CAD build for the part. Positions are in the model's coordinates, mm. Face numbers are marked on the shaded views. A direction names the side the tool comes from. Coordinates: 2 decimals unless noted, no trailing zeros. Write each loop counter-clockwise with the first axis right and the second up, starting at its lowest first coordinate (ties: lowest second). Pieces come first, ordered by that corner, then holes. Notation, with made-up numbers: (-20.5, 61) - (11.5, 61) arc R27 ccw to (11.5, 78) - close; hole circle Ø5 at (62.25, 16). An arc over 180 degrees is marked (long way). Answer in a Markdown table with one row per item. Add a question column.
Q1. Band-saw the part on D-D (x = -16). List the corners of the cut face in (y, z).
Q2. Band-saw the part on A-A (y = -54). List the corners of the cut face in (x, z).
Q3. Drill centre lines: line 1 along Z through (x, y) = (25, 51); line 2 along Y through (x, z) = (-34, -65); line 3 along Y through (x, z) = (-35, -37). Where is each one in solid material? Low to high. Write a range as from..to.
Q4. 3-axis set-ups, long thin cutter, end or side, ignore diameter. For the marked faces 1 and 2: which of +Z, -Z, +X, -X, +Y, -Y reach the whole face in a straight line?
Q5. Band-saw the part on B-B (x = -39). List the corners of the cut face in (y, z).
Q6. Band-saw the part on C-C (z = -28.5). List the corners of the cut face in (x, y), and give its area (3 significant figures).
Q7. Pin check, flat tips, straight feed: pin 1 (6 mm diameter, centred on x = -14.5, y = -24, fed in from -Z); pin 2 (2.5 mm diameter, centred on x = 34.5, y = 59.5, fed in from -Z); pin 3 (3 mm diameter, centred on x = 29.5, z = -61.5, fed in from -Y); pin 4 (9.5 mm diameter, centred on x = -37, y = -56.5, fed in from -Z). Stop position of each tip, or through.
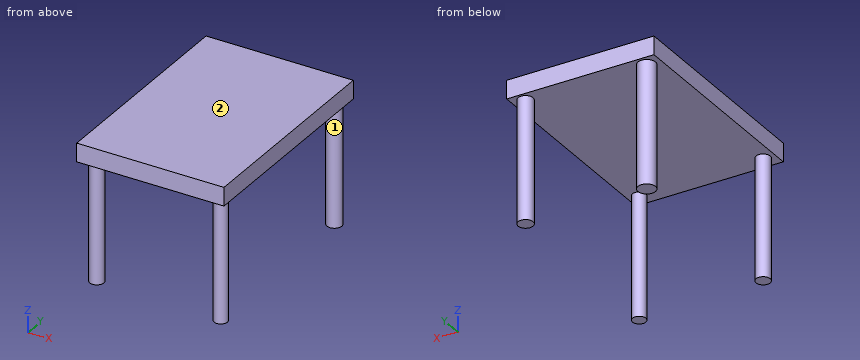
```python
from build123d import *

# Parameters (mm, degrees)
F0_W     = 89.114376
F0_H     = 129.904926
F1_DEPTH = 11.176
F2_R     = 5.277651
F6_DEPTH = 74.422
F3_R     = 4.552344
F7_DEPTH = 74.168
F4_R     = 4.294458
F8_DEPTH = 73.406
F5_R     = 4.020045
F9_DEPTH = 74.422


with BuildPart() as f1:
    # F0 (on Top) → F1 (new body)
    with BuildSketch(Plane.XY):
        Rectangle(F0_W, F0_H)
    extrude(amount=F1_DEPTH)

    # F2 (on Top) → F6 (join)
    with BuildSketch(Plane.XY):
        with Locations((-36.073875, 58.119018)):
            Circle(F2_R)
    extrude(amount=-F6_DEPTH)

    # F3 (on face) → F7 (join)
    with BuildSketch(Plane(origin=(0, 0, 0), x_dir=(1, 0, 0), z_dir=(0, 0, -1))):
        with Locations((36.690522, -59.043989)):
            Circle(F3_R)
    extrude(amount=F7_DEPTH)

    # F4 (on Top) → F8 (join)
    with BuildSketch(Plane.XY):
        with Locations((-37.615493, -56.269072)):
            Circle(F4_R)
    extrude(amount=-F8_DEPTH)

    # F5 (on Top) → F9 (join)
    with BuildSketch(Plane.XY):
        with Locations((37.615493, -56.577403)):
            Circle(F5_R)
    extrude(amount=-F9_DEPTH)


solid = f1.part
```
Checked values:
| question | item | result |
|---|---|---|
| 1 | outline | (-64.95, 0) - (64.95, 0) - (64.95, 11.18) - (-64.95, 11.18) - close |
| 2 | outline | (-44.56, 0) - (-41.26, 0) - (-41.26, -73.41) - (-33.97, -73.41) - (-33.97, 0) - (34.53, 0) - (34.53, -74.42) - (40.7, -74.42) - (40.7, 0) - (44.56, 0) - (44.56, 11.18) - (-44.56, 11.18) - close |
| 3 | line 1 | z = 0..11.18 |
| 3 | line 2 | y = -58.59..-53.95, 53.27..62.97 |
| 3 | line 3 | y = -59.68..-52.86, 52.95..63.29 |
| 4 | face 1 | -Z |
| 4 | face 2 | +Z, +X, -X, +Y, -Y |
| 5 | outline | (-64.95, 0) - (-60.33, 0) - (-60.33, -73.41) - (-52.2, -73.41) - (-52.2, 0) - (53.73, 0) - (53.73, -74.42) - (62.51, -74.42) - (62.51, 0) - (64.95, 0) - (64.95, 11.18) - (-64.95, 11.18) - close |
| 6 | outline | circle Ø8.59 at (-37.62, -56.27); circle Ø10.56 at (-36.07, 58.12); circle Ø9.1 at (36.69, 59.04); circle Ø8.04 at (37.62, -56.58) |
| 6 | area | 261 mm² |
| 7 | pin 1 | stops at z = 0 |
| 7 | pin 2 | stops at z = -74.17 |
| 7 | pin 3 | passes through |
| 7 | pin 4 | stops at z = -73.41 |
